```python
from build123d import *

# Parameters (mm, degrees)
SKETCH1_R           = 2.001
SKETCH1_R_2         = 2.5
SKETCH1_R_3         = 2
BOSS_EXTRUDE2_DEPTH = 4


with BuildPart() as part:
    # Sketch1 → Boss-Extrude2 (new body)
    with BuildSketch(Plane.XY):
        with BuildLine():
            Line((249.889094902, -24.965497133), (254.003864049, -33.092166198))
            ThreePointArc((254.003864049, -33.092166198), (255.292000843, -36.604410668), (255.729349518, -40.319768492))
            Line((255.729349518, -40.319768492), (255.729349518, -44.113946135))
            ThreePointArc((255.729349518, -44.113946135), (252.381328024, -53.908201589), (243.738419531, -59.60353482))
            Line((243.738419531, -59.60353482), (195.72651514, -72.030145369))
            ThreePointArc((195.72651514, -72.030145369), (193.025606236, -73.809937003), (191.979349518, -76.870641833))
            Line((191.979349518, -76.870641833), (191.979349518, -78))
            ThreePointArc((191.979349518, -78), (193.443815613, -81.535533906), (196.979349518, -83))
            Line((196.979349518, -83), (241.979349518, -83))
            ThreePointArc((241.979349518, -83), (263.192552954, -74.213203436), (271.979349518, -53))
            Line((271.979349518, -53), (271.979349518, -20))
            ThreePointArc((271.979349518, -20), (277.837213895, -5.857864376), (291.979349518, 0))
            Line((291.979349518, 0), (322.729349518, 0))
            ThreePointArc((322.729349518, 0), (324.850669862, 0.878679656), (325.729349518, 3))
            Line((325.729349518, 3), (325.729349518, 7))
            ThreePointArc((325.729349518, 7), (324.850669862, 9.121320344), (322.729349518, 10))
            Line((322.729349518, 10), (238.729349518, 10))
            ThreePointArc((238.729349518, 10), (236.608029175, 9.121320344), (235.729349518, 7))
            Line((235.729349518, 7), (235.729349518, 6.819768492))
            ThreePointArc((235.729349518, 6.819768492), (236.166698194, 3.104410668), (237.454834988, -0.407833802))
            Line((237.454834988, -0.407833802), (238.081894478, -1.646276295))
            ThreePointArc((238.081894478, -1.646276295), (237.961390247, -4.571220464), (235.406315161, -6))
            Line((235.406315161, -6), (194.978349518, -6))
            ThreePointArc((194.978349518, -6), (192.857736282, -6.878386763), (191.979349518, -8.999))
            Line((191.979349518, -8.999), (191.979349518, -11.001))
            ThreePointArc((191.979349518, -11.001), (192.857736282, -13.121613237), (194.978349518, -14))
            Line((194.978349518, -14), (232.045951739, -14))
            ThreePointArc((232.045951739, -14), (242.517578705, -16.960486255), (249.889094902, -24.965497133))
        make_face()
        with Locations((226.979349518, -10)):
            Circle(SKETCH1_R, mode=Mode.SUBTRACT)
        with Locations((196.979349518, -10)):
            Circle(SKETCH1_R, mode=Mode.SUBTRACT)
        with Locations((201.979349518, -77.435320916)):
            Circle(SKETCH1_R_2, mode=Mode.SUBTRACT)
        with Locations((241.979349518, -77.435320916)):
            Circle(SKETCH1_R_2, mode=Mode.SUBTRACT)
        with Locations((255.729349518, 5)):
            Circle(SKETCH1_R_3, mode=Mode.SUBTRACT)
        with Locations((288.229349518, 5)):
            Circle(SKETCH1_R_3, mode=Mode.SUBTRACT)
        with Locations((320.729349518, 5)):
            Circle(SKETCH1_R_3, mode=Mode.SUBTRACT)
    extrude(amount=BOSS_EXTRUDE2_DEPTH)


solid = part.part
```
Here's how the part is built. I have some questions about the finished solid (model axes, mm). A direction names the side the tool comes from. Round coordinates to 2 decimals unless told otherwise and drop trailing zeros. Write each loop counter-clockwise with the first axis right and the second up, starting at its lowest first coordinate (ties: lowest second). Pieces come first, ordered by that corner, then holes. Notation, with made-up numbers: M 48.25,71 L 66.25,71 A28 ccw 66.25,90 Z; hole C 10,-12 d11. An arc over 180 degrees is marked long. Answer as CSV lines item,"result". Start each with the question number.
1. Suppose I cut it at B-B on z = 2.55. Count the separate pieces of the cut face and the enclosed holes in it, then the cut area to 3 significant figures.
2. I'm going to push flat-ended pins straight in: pin 1 Ø1.2 at (y, z) = (-44, 1.5) entering from +X; pin 2 Ø3 at (x, y) = (288.23, 5) entering from +Z; pin 3 Ø1.2 at (x, z) = (302, 1) entering from -Y; pin 4 Ø1 at (x, z) = (281, 2) entering from -Y. Where does each tip first touch, or does it pass through?
3. Suppose I cut it at D-D on y = -57. Write out the boundary of the cut face in (x, z), then the cut area to 3 significant figures.
4. Suppose I cut it at A-A on y = 5. Write out the boundary of the cut face in (x, z), then the cut area to 3 significant figures.
5. Thinking about a two-plate mould opening in X: for faces 1 (the flat face through (271.979, -37, 2)), 2 (the cylindrical face through (192.881, -6.855, 1.972)), 3 (the cylindrical face through (318.73, 5.09, 1.97)), which applies, released by +X, released by -X, zero draft, split by the parting line, or undercut?
6. On a 3-axis mill with a long thin cutter (end or side, diameter ignored), from which of +Z, -Z, +X, -X, +Y, -Y can I reach the whole of each face in a straight line? I mean faces 4 (the cylindrical face through (195.391, -11.218, 1.972)), 5 (the cylindrical face through (192.835, -13.098, 1.972)). Say none if no direction works.
7. I need wall thicknesses on probe 1 along Y at (x, z) = (203, 2.25); probe 2 along Y at (x, z) = (221, 3); probe 3 along Y at (x, z) = (248, 2.75). Which ranges of each line are inside material? Lowest first, please.
8. Suppose I cut it at C-C on y = -39. Write out the boundary of the cut face in (x, z), then the cut area to 3 significant figures.
Check result:
1,separate pieces,"1"
1,enclosed holes,"7"
1,area,"3,980 mm2"
2,pin 1,"stops at x = 271.98"
2,pin 2,"passes through"
2,pin 3,"stops at y = 0"
2,pin 4,"stops at y = -3.62"
3,outline,"M 249.21,0 L 271.71,0 L 271.71,4 L 249.21,4 Z"
3,area,"90.0 mm2"
4,outline,"M 235.83,0 L 253.73,0 L 253.73,4 L 235.83,4 Z; M 257.73,0 L 286.23,0 L 286.23,4 L 257.73,4 Z; M 290.23,0 L 318.73,0 L 318.73,4 L 290.23,4 Z; M 322.73,0 L 325.73,0 L 325.73,4 L 322.73,4 Z"
4,area,"312 mm2"
5,face 1,"released by +X"
5,face 2,"released by -X"
5,face 3,"undercut"
6,face 4,"+Z, -Z"
6,face 5,"+Z, -Z, -X"
7,probe 1,"y = -83 to -79.72, -75.15 to -70.15, -14 to -6"
7,probe 2,"y = -83 to -65.49, -14 to -6"
7,probe 3,"y = -82.39 to -57.81, -21.94 to 10"
8,outline,"M 255.67,0 L 271.98,0 L 271.98,4 L 255.67,4 Z"
8,area,"65.2 mm2"
